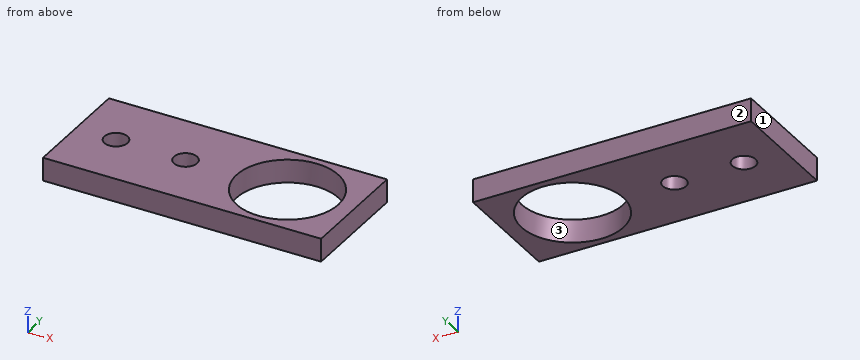
```python
from build123d import *

# Parameters (mm, degrees)
SKETCH1_W           = 60
SKETCH1_H           = 25
SKETCH1_R           = 2.5
SKETCH1_R_2         = 11
BOSS_EXTRUDE2_DEPTH = 5


with BuildPart() as part:
    # Sketch1 → Boss-Extrude2 (new body)
    with BuildSketch(Plane.XY):
        Rectangle(SKETCH1_W, SKETCH1_H)
        with Locations((-21.359853693, 0)):
            Circle(SKETCH1_R, mode=Mode.SUBTRACT)
        with Locations((15.644174596, 0)):
            Circle(SKETCH1_R_2, mode=Mode.SUBTRACT)
        with Locations((-6.359853693, 0)):
            Circle(SKETCH1_R, mode=Mode.SUBTRACT)
    extrude(amount=BOSS_EXTRUDE2_DEPTH)


solid = part.part
```
Verification items for the finished model (mm, model axes). Face numbers are marked on the shaded views. Give positions to 0.01 mm unless a question says otherwise; leave off trailing zeros. Order: outer loops, then holes, each group sorted by start corner. A loop starts at its lowest first (then second) coordinate and runs counter-clockwise, first axis right, second up. Notation, with made-up numbers: M 38.25,1 L 52.25,1 A8 ccw 52.25,7 Z; hole C 50.5,82 d2. An arc over 180 degrees is marked long. Return JSON: item names as keys, results as strings. Group by question number.
1) Section check C-C on y = -5.75. Record the cut outline in (x, z), and give its area (3 significant figures).
2) Mould release check, pull along X, two halves, no side actions. Record for the marked faces 1, 2 and 3: pulls with the +X half, pulls with the -X half, needs draft (parallel to the pull), parting line crosses it, or undercut.
3) Section check B-B on z = 3.2. Record the cut outline in (x, y).
4) Scan lines: line 1 (X direction, y = 1, z = 2.15); line 2 (Y direction, x = 15.5, z = 4.75); line 3 (Y direction, x = -22, z = 0.95). Record each from-to range of solid material in increasing order.
5) Section check A-A on y = 0. Record the cut outline in (x, z), and give its area (3 significant figures).
6) Go/stop test with a flat-tipped pin: pin 1 Ø13 at (x, y) = (15.64, 0) entering from -Z. Record where the tip stops, or that it passes through.
7) Section check D-D on y = 4.25. Record the cut outline in (x, z).
Answer block:
{
 "1": {"outline": "M -30,0 L 6.27,0 L 6.27,5 L -30,5 Z; M 25.02,0 L 30,0 L 30,5 L 25.02,5 Z", "area": "206 mm^2"},
 "2": {"face 1": "pulls with the -X half", "face 2": "needs draft", "face 3": "undercut"},
 "3": {"outline": "M -30,-12.5 L 30,-12.5 L 30,12.5 L -30,12.5 Z; hole C -21.36,0 d5; hole C -6.36,0 d5; hole C 15.64,0 d22"},
 "4": {"line 1": "x = -30 to -23.65, -19.07 to -8.65, -4.07 to 4.69, 26.6 to 30", "line 2": "y = -12.5 to -11, 11 to 12.5", "line 3": "y = -12.5 to -2.42, 2.42 to 12.5"},
 "5": {"outline": "M -30,0 L -23.86,0 L -23.86,5 L -30,5 Z; M -18.86,0 L -8.86,0 L -8.86,5 L -18.86,5 Z; M -3.86,0 L 4.64,0 L 4.64,5 L -3.86,5 Z; M 26.64,0 L 30,0 L 30,5 L 26.64,5 Z", "area": "140 mm^2"},
 "6": {"pin 1": "passes through"},
 "7": {"outline": "M -30,0 L 5.5,0 L 5.5,5 L -30,5 Z; M 25.79,0 L 30,0 L 30,5 L 25.79,5 Z"}
}
